Source: CAD feature listing. Evaluate the final solid. Frame: model axes, mm. Face numbers are marked on the shaded views. A direction names the side the tool comes from. Give positions to 0.01 mm unless a question says otherwise; leave off trailing zeros. Loops run counter-clockwise (first coordinate to the right, second up) from the corner with the lowest first, then second, coordinate; pieces in that order, holes last. Notation, with made-up numbers: (25.25, 19) -> (79.25, 19) arc R10 cw to (79.25, 32) -> close; hole circle Ø5 at (31.25, 77.25). An arc over 180 degrees is marked (long way). Put each result on its own line as item: value.
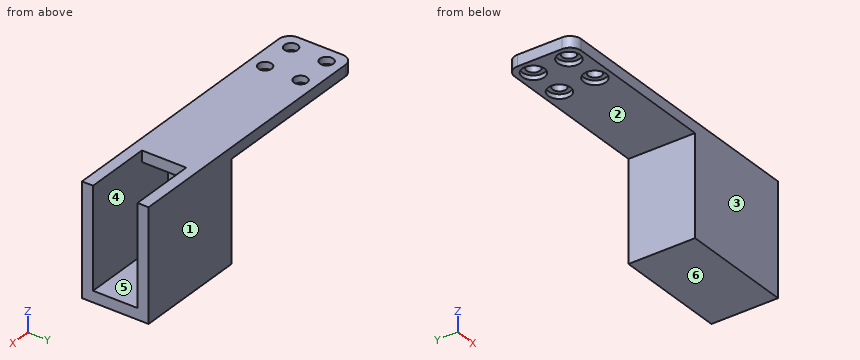
Autodesk Fusion 360 part; units mm, degrees
sketch "Sketch1" plane through (0, 0, 0) normal (0, 0, 1) x (1, 0, 0)
  line L0 (0, 0) -> (51, 0)
  line L1 (51, 0) -> (51, -30)
  line L2 (51, -30) -> (0, -30)
  line L3 (0, -30) -> (0, 0)
  dimension "d1" = 51
  dimension "d2" = 30
extrude "Extrude1" add sketch "Sketch1" along normal blind 50
sketch "Sketch2" plane through (51, 0, 0) normal (1, 0, 0) x (0, 1, 0)
  line L0 (-30, 0) -> (0, 0)
  line L1 (0, 0) -> (0, 50)
  line L2 (0, 50) -> (-30, 50)
  line L3 (-30, 50) -> (-30, 0)
  line L4 (-5, 5) -> (-25, 5)
  line L5 (-25, 5) -> (-25, 45)
  line L6 (-25, 45) -> (-5, 45)
  line L7 (-5, 45) -> (-5, 5)
  dimension "d5" = 20
  dimension "d6" = 40
extrude "Extrude2" cut sketch "Sketch2" against normal blind 46 contours L4 L5 L6 L7
sketch "Sketch3" plane through (0, 0, 50) normal (0, 0, 1) x (-1, 0, 0)
  line L0 (0, 30) -> (-51, 30)
  line L1 (-51, 30) -> (-51, 0)
  line L2 (-51, 0) -> (0, 0)
  line L3 (0, 0) -> (0, 30)
  line L4 (-51, 5) -> (-21, 5)
  line L5 (-21, 5) -> (-21, 25)
  line L6 (-21, 25) -> (-51, 25)
  line L7 (-51, 25) -> (-51, 5)
  dimension "d9" = 30
  dimension "d10" = 20
extrude "Extrude3" cut sketch "Sketch3" against normal blind 6 contours L1 L4 L5 L6 L7
sketch "Sketch4" plane through (0, 0, 50) normal (0, 0, 1) x (-1, 0, 0)
  line L0 (-51, 25) -> (-21, 25)
  line L1 (-21, 25) -> (-21, 5)
  line L2 (-21, 5) -> (-51, 5)
  line L3 (-51, 5) -> (-51, 0)
  line L4 (-51, 0) -> (0, 0)
  line L5 (0, 0) -> (0, 30)
  line L6 (0, 30) -> (-51, 30)
  line L7 (-51, 30) -> (-51, 25)
  line L8 (0, 0) -> (75, 0)
  line L9 (75, 0) -> (75, 30)
  line L10 (75, 30) -> (0, 30)
  line L11 (0, 30) -> (0, 0)
  dimension "d13" = 75
  dimension "d14" = 30
extrude "Extrude4" add sketch "Sketch4" against normal blind 5 contours L5 L8 L9 L10 L11
sketch "Sketch5" plane through (0, 0, 50) normal (0, 0, 1) x (-1, 0, 0)
  line L0 (-51, 25) -> (-21, 25)
  line L1 (-21, 25) -> (-21, 5)
  line L2 (-21, 5) -> (-51, 5)
  line L3 (-51, 5) -> (-51, 0)
  line L4 (-51, 0) -> (75, 0)
  line L5 (75, 0) -> (75, 30)
  line L6 (75, 30) -> (-51, 30)
  line L7 (-51, 30) -> (-51, 25)
  circle A0 centre (68, 7) radius 3
  circle A1 centre (68, 23) radius 3
  circle A2 centre (52, 7) radius 3
  circle A3 centre (52, 23) radius 3
  dimension "d17" = 6
  dimension "d18" = 6
  dimension "d19" = 6
  dimension "d20" = 6
extrude "Extrude5" cut sketch "Sketch5" against normal blind 5 contours A0 | A1 | A2 | A3
sketch "Sketch6" plane through (0, 0, 45) normal (0, 0, -1) x (1, 0, 0)
  circle A0 centre (-68, 23) radius 3
  circle A1 centre (-68, 7) radius 3
  circle A2 centre (-52, 23) radius 3
  circle A3 centre (-52, 7) radius 3
  line L0 (0, 0) -> (0, 30)
  line L1 (0, 30) -> (-75, 30)
  line L2 (-75, 30) -> (-75, 0)
  line L3 (-75, 0) -> (0, 0)
  circle A4 centre (-68, 23) radius 5
  circle A5 centre (-52, 23) radius 5
  circle A6 centre (-68, 7) radius 5
  circle A7 centre (-52, 7) radius 5
  dimension "d23" = 10
  dimension "d24" = 10
  dimension "d25" = 10
  dimension "d26" = 10
extrude "Extrude6" cut sketch "Sketch6" against normal blind 2 contours A4 | A5 | A6 | A7
fillet "Fillet1" radius 5 2 edges at (-75, -30, 47.5) (-75, 0, 47.5)
(1) Draft query along Z for the marked faces 3, 4, 5 and 6. Return one class per face: released by +Z, released by -Z, zero draft, split by the parting line, or undercut.
Calculated:
face 3: zero draft
face 4: undercut
face 5: undercut
face 6: released by -Z
(2) First-contact query: P1, Ø9, axis at x = -68, y = -7, coming from the -Z side; P2, Ø11.5, axis at x = -52, y = -7, coming from the -Z side; P3, Ø7, axis at x = -52, y = -23, coming from the +Z side; P4, Ø10, axis at x = 36, y = -18.5, coming from the +Z side. Flat tips, straight axial feed; report the tip coordinate or a pass-through.
Calculated:
P1: stops at z = 47
P2: stops at z = 45
P3: stops at z = 50
P4: stops at z = 5
(3) Reachability of the marked faces 1 and 2 from +Z, -Z, +X, -X, +Y, -Y: full face, straight path, thin tool, end or side. Return the list, or none.
Calculated:
face 1: +Z, -Z, +X, -X, +Y
face 2: -Z, -X, +Y, -Y
(4) Section D-D on z = 22. Return loops of the section in (x, y).
Calculated:
outline: (0, -30) -> (51, -30) -> (51, -25) -> (5, -25) -> (5, -5) -> (51, -5) -> (51, 0) -> (0, 0) -> close
(5) Section B-B on x = -52. Return loops of the section in (y, z), then the cut area to 3 significant figures.
Calculated:
outline: (-30, 45) -> (-28, 45) -> (-28, 47) -> (-26, 47) -> (-26, 50) -> (-30, 50) -> close; (-20, 47) -> (-18, 47) -> (-18, 45) -> (-12, 45) -> (-12, 47) -> (-10, 47) -> (-10, 50) -> (-20, 50) -> close; (-4, 47) -> (-2, 47) -> (-2, 45) -> (0, 45) -> (0, 50) -> (-4, 50) -> close
area: 74.0 mm²
(6) Section C-C on x = 28. Return loops of the section in (y, z).
Calculated:
outline: (-30, 0) -> (0, 0) -> (0, 50) -> (-5, 50) -> (-5, 5) -> (-25, 5) -> (-25, 50) -> (-30, 50) -> close
(7) Section A-A on y = -7. Return loops of the section in (x, z), then the cut area to 3 significant figures.
Calculated:
outline: (-75, 45) -> (-73, 45) -> (-73, 47) -> (-71, 47) -> (-71, 50) -> (-75, 50) -> close; (-65, 47) -> (-63, 47) -> (-63, 45) -> (-57, 45) -> (-57, 47) -> (-55, 47) -> (-55, 50) -> (-65, 50) -> close; (-49, 47) -> (-47, 47) -> (-47, 45) -> (0, 45) -> (0, 0) -> (51, 0) -> (51, 5) -> (5, 5) -> (5, 45) -> (21, 45) -> (21, 50) -> (-49, 50) -> close
area: 859 mm²
(8) Line query: probe 1 along X at (y, z) = (-23, 46.2); probe 2 along X at (y, z) = (-7, 48); probe 3 along Y at (x, z) = (-52, 48.8). Output: solid intervals per line, ascending. Write a range as from..to.
Calculated:
probe 1: x = -75..-73, -63..-57, -47..21
probe 2: x = -75..-71, -65..-55, -49..21
probe 3: y = -30..-26, -20..-10, -4..0
